```python
from build123d import *

# Parameters (mm, degrees)
SKETCH1_R           = 3.75
BOSS_EXTRUDE1_DEPTH = 1
SKETCH2_R           = 1.875
BOSS_EXTRUDE2_DEPTH = 20
SKETCH3_R           = 2.375
BOSS_EXTRUDE3_DEPTH = 1
SKETCH4_W           = 0.75
SKETCH4_H           = 8
CUT_EXTRUDE1_DEPTH  = 7.5
CUT_EXTRUDE2_START  = -10
CUT_EXTRUDE2_DEPTH  = 10


with BuildPart() as part:
    # Sketch1 → Boss-Extrude1 (new body)
    with BuildSketch(Plane(origin=(0, 0, 0), x_dir=(1, 0, 0), z_dir=(0, 1, 0))):
        with Locations(Location((0, 0, 0), (0, 0, 270))):
            Circle(SKETCH1_R)
    extrude(amount=BOSS_EXTRUDE1_DEPTH)

    # Sketch2 → Boss-Extrude2 (add)
    with BuildSketch(Plane(origin=(0, 1, 0), x_dir=(1, 0, 0), z_dir=(0, 1, 0))):
        with Locations(Location((0, 0, 0), (0, 0, 270))):
            Circle(SKETCH2_R)
    extrude(amount=BOSS_EXTRUDE2_DEPTH)

    # Sketch3 → Boss-Extrude3 (add)
    with BuildSketch(Plane(origin=(0, 21, 0), x_dir=(1, 0, 0), z_dir=(0, 1, 0))):
        with Locations(Location((0, 0, 0), (0, 0, 270))):
            Circle(SKETCH3_R)
    extrude(amount=BOSS_EXTRUDE3_DEPTH)

    # Sketch4 → Cut-Extrude1 (cut)
    with BuildSketch(Plane(origin=(0, 22, 0), x_dir=(1, 0, 0), z_dir=(0, 1, 0))):
        Rectangle(SKETCH4_W, SKETCH4_H)
    extrude(amount=-CUT_EXTRUDE1_DEPTH, mode=Mode.SUBTRACT)

    # Sketch5 → Cut-Extrude2 (cut)
    with BuildSketch(Plane(origin=(0, 22, 0), x_dir=(1, 0, 0), z_dir=(0, 1, 0)).offset(CUT_EXTRUDE2_START)):
        with BuildLine():
            Line((1.803285686, -1.545569712), (0.375, -1.837117307))
            Line((0.375, -1.837117307), (0.375, -2.34520788))
            ThreePointArc((0.375, -2.34520788), (1.160210081, -2.072326607), (1.803285686, -1.545569712))
        make_face()
        with BuildLine():
            Line((0.375, 2.34520788), (0.375, 1.837117307))
            Line((0.375, 1.837117307), (1.803285686, 1.545569712))
            ThreePointArc((1.803285686, 1.545569712), (1.160210081, 2.072326607), (0.375, 2.34520788))
        make_face()
        with BuildLine():
            Line((-1.803285686, 1.545569712), (-0.375, 1.837117307))
            Line((-0.375, 1.837117307), (-0.375, 2.34520788))
            ThreePointArc((-0.375, 2.34520788), (-1.160210081, 2.072326607), (-1.803285686, 1.545569712))
        make_face()
        with BuildLine():
            Line((-0.375, -2.34520788), (-0.375, -1.837117307))
            Line((-0.375, -1.837117307), (-1.803285686, -1.545569712))
            ThreePointArc((-1.803285686, -1.545569712), (-1.160210081, -2.072326607), (-0.375, -2.34520788))
        make_face()
    extrude(amount=CUT_EXTRUDE2_DEPTH, mode=Mode.SUBTRACT)


solid = part.part
```
Here's how the part is built. I have some questions about the finished solid (model axes, mm). A direction names the side the tool comes from. Round coordinates to 2 decimals unless told otherwise and drop trailing zeros. Order: outer loops, then holes, each group sorted by start corner. A loop starts at its lowest first (then second) coordinate and runs counter-clockwise, first axis right, second up. Notation, with made-up numbers: M 2.25,79.25 L 56.25,79.25 A11 cw 56.25,97.25 Z; hole C 9,83.5 d11. An arc over 180 degrees is marked long. Answer in a Markdown table with one row per item.
Item 1: Thinking about a two-plate mould opening in Y: for faces 6 (the face through (-0.72, 10.86, 1.73)), 7 (the face through (0, 0, 0)), 8 (the face through (-2.375, 21.493, -0.024)), 9 (the face through (-2.04, 21, -0.01)), which applies, +Y half, -Y half, draft (parallel to the pull), parting line (faces both ways), or undercut?
A:
| item | result |
|---|---|
| face 6 | undercut |
| face 7 | -Y half |
| face 8 | draft |
| face 9 | undercut |
Item 2: I'm going to push flat-ended pins straight in: pin 1 (1 mm diameter, centred on x = -2, y = 10, fed in from -Z) (3 decimals); pin 2 (1.1 mm diameter, centred on y = 20, z = 0, fed in from -X) (3 decimals); pin 3 (1.5 mm diameter, centred on x = 1, y = 19, fed in from +Z); pin 4 (2 mm diameter, centred on x = -1.5, z = -1, fed in from -Y). Where does each tip first touch, or does it pass through?
A:
| item | result |
|---|---|
| pin 1 | stops at z = -1.125 |
| pin 2 | stops at x = -1.875 |
| pin 3 | stops at z = 1.84 |
| pin 4 | stops at y = 0 |
Item 3: Imagine slicing it at D-D, the plane y = 10.25. Write out the boundary of the cut face in (x, z) (3 decimals), and give its area (3 significant figures).
A:
| item | result |
|---|---|
| outline | C 0,0 d3.75 |
| area | 11.0 mm2 |
Item 4: Imagine slicing it at B-B, the plane y = 17.5. Write out the boundary of the cut face in (x, z) (3 decimals), and give its area (3 significant figures).
A:
| item | result |
|---|---|
| outline | M -0.375,-1.837 L -0.375,1.837 A1.875 ccw Z; M 0.375,-1.837 A1.875 ccw 0.375,1.837 Z |
| area | 8.25 mm2 |
Item 5: Imagine slicing it at C-C, the plane x = -1.5. Write out the boundary of the cut face in (y, z) (3 decimals).
A:
| item | result |
|---|---|
| outline | M 0,-3.437 L 1,-3.437 L 1,-1.125 L 21,-1.125 L 21,-1.607 L 22,-1.607 L 22,1.607 L 21,1.607 L 21,1.125 L 1,1.125 L 1,3.437 L 0,3.437 Z |
Item 6: Imagine slicing it at A-A, the plane z = 0. Write out the boundary of the cut face in (x, y) (3 decimals), and give its area (3 significant figures).
A:
| item | result |
|---|---|
| outline | M -3.75,0 L 3.75,0 L 3.75,1 L 1.875,1 L 1.875,21 L 2.375,21 L 2.375,22 L 0.375,22 L 0.375,14.5 L -0.375,14.5 L -0.375,22 L -2.375,22 L -2.375,21 L -1.875,21 L -1.875,1 L -3.75,1 Z |
| area | 81.6 mm2 |
Item 7: For faces 1 (the face through (1.1, 21.49, 1.69)), 2 (the face through (-1.079, 21.493, 1.693)), 3 (the face through (2.05, 21, 0.13)), 4 (the face through (-1.1, 21.49, -1.69)), 5 (the face through (0.375, 18, 0)), which set-ups out of +Z, -Z, +X, -X, +Y, -Y let a thin tool reach every point of the face, with its end or its side?
A:
| item | result |
|---|---|
| face 1 | +Z, +X, +Y |
| face 2 | +Z, -X, +Y |
| face 3 | +X |
| face 4 | -Z, -X, +Y |
| face 5 | +Z, -Z, +Y |
Item 8: If I drill on L1, parallel to Y at x = -2, z = -0.75; L2, parallel to Y at x = -2.75, z = -2.5; L3, parallel to X at y = 8, z = -0.5, over which ranges is the centre line in solid material (lowest first)? Write a range as from..to.
A:
| item | result |
|---|---|
| L1 | y = 0..1, 21..22 |
| L2 | y = 0..1 |
| L3 | x = -1.81..1.81 |
